Input: part model. Units: mm. Frame: model coordinates. A direction names the side the tool comes from. Give positions to 0.01 mm unless a question says otherwise; leave off trailing zeros. Order: outer loops, then holes, each group sorted by start corner. A loop starts at its lowest first (then second) coordinate and runs counter-clockwise, first axis right, second up. Notation, with made-up numbers: M 88,-37.5 L 109,-37.5 A24 ccw 109,-12.5 Z; hole C 19,8 d2. An arc over 180 degrees is marked long. Use a Markdown table: item, result.
Autodesk Inventor part; units mm, degrees
ref_plane "YZ Plane" through (0, 0, 0) normal (1, 0, 0) x (0, 1, 0)
ref_plane "XZ Plane" through (0, 0, 0) normal (0, 1, 0) x (-1, 0, 0)
ref_plane "XY Plane" through (0, 0, 0) normal (0, 0, 1) x (1, 0, 0)
sketch "Sketch1" plane through (0, 0, 0) normal (1, 0, 0) x (0, 1, 0)
  line L0 (-22.6931, 110) -> (55.0359, 110)
  line L1 (55, -110) -> (-22.6931, -110)
  line L2 (-62.7298, 0) -> (-22.6931, -110)
  line L3 (-62.7298, 0) -> (-22.6931, 110)
  line L4 (-57.4089, 0) -> (-19.449, -104.2938)
  line L5 (-14.4482, -105) -> (55, -105)
  line L6 (55.0359, 105) -> (-14.4122, 105)
  line L7 (-19.449, 104.2938) -> (-57.4089, 0)
  line L8 (55.0034, 17.6855) -> (-14.4593, 17.6855)
  line L9 (55.0034, 22.5) -> (-14.4456, 22.5496)
  line L10 (55, -52.5) -> (-14.449, -52.5)
  line L11 (55, -47.6855) -> (-14.449, -47.7352)
  line L12 (-60.6224, -5.7899) -> (-60, -7.5)
  line L13 (-60.6224, 5.7899) -> (-60, 7.5)
  line L14 (-14.4122, 105) -> (-14.4122, 68.1255)
  line L15 (-14.4456, 59.4672) -> (-14.4456, 22.5496)
  line L16 (-19.449, 104.2938) -> (-19.449, 68.1255)
  line L17 (-14.4593, 17.6855) -> (-14.4593, -10.5317)
  line L18 (-14.449, -19.4683) -> (-14.449, -47.7352)
  line L19 (-19.4705, 59.4672) -> (-19.4705, -10.5317)
  line L20 (-14.449, -52.5) -> (-14.449, -74.4672)
  line L21 (-14.4482, -83.1255) -> (-14.4482, -105.0928)
  line L22 (-19.4499, -19.4683) -> (-19.4499, -74.4672)
  line L23 (-19.449, -83.1255) -> (-19.449, -104.2938)
  line L24 (-19.449, -74.4672) -> (-19.4499, -74.4672)
  line L25 (-14.4593, -83.1255) -> (-14.4482, -83.1255)
  line L26 (-19.4499, -19.4683) -> (-19.449, -19.4683)
  line L27 (-19.4705, -10.5317) -> (-19.449, -10.5317)
  line L28 (-14.4122, 68.1255) -> (-14.4125, 68.1255)
  line L29 (-19.4705, 59.4672) -> (-19.449, 59.4672)
  line L30 (55.0359, 105) -> (55.0359, 110)
  line L31 (55.0034, 22.5) -> (55.0034, 17.6855)
  line L32 (55, -47.6855) -> (55, -52.5)
  line L33 (55, -105) -> (55, -110)
  line L34 (-19.449, -91.3967) -> (-19.449, 76.5553)
  line L35 (-14.4122, 69.213) -> (-14.4225, 22.5496)
  line L36 (-14.4236, 17.6855) -> (-14.438, -47.7351)
  line L37 (-14.439, -52.5) -> (-14.4482, -94.1091)
  point P0 (0, 0)
extrude "Extrusion1" add sketch "Sketch1" along normal blind 160
sketch "Sketch2" plane through (0, -14.4236, 17.6855) normal (0, 1, -0.0002) x (1, 0, 0)
  circle A0 centre (80, 33.4744) radius 10
  circle A1 centre (80, 98.5003) radius 10
  circle A2 centre (80, -44.9284) radius 10
  point P0 (0, 17.6824)
  dimension "d24" = 20
  dimension "d25" = 20
  dimension "d26" = 20
extrude "Extrusion2" cut sketch "Sketch2" against normal blind 6
sketch "Sketch3" plane through (0, -22.6931, -110) normal (0, -0.9397, -0.342) x (1, 0, 0)
  point P0 (0, 95.6047)
sketch "Sketch4" plane through (0, -22.6931, -110) normal (0, -0.9397, -0.342) x (1, 0, 0)
  line L0 (0, 117.1568) -> (160, 117.1568)
  circle A0 centre (80, 117.1568) radius 7.5
  point P0 (0, 95.6047)
  dimension "d29" = 15
extrude "Extrusion3" cut sketch "Sketch4" against normal blind 10
sketch "Sketch5" plane through (0, 0, 0) normal (-1, 0, 0) x (0, 0, 1)
  line L0 (-110, -22.6931) -> (-110, 55)
  line L1 (-110, 55) -> (109.7253, 55)
  line L2 (109.7253, 55) -> (109.7253, -62.9244)
  line L3 (109.7253, -62.9244) -> (-110, -62.9244)
  line L4 (-110, -62.9244) -> (-110, 55)
  point P0 (0, 0)
extrude "Extrusion4" add sketch "Sketch5" along normal blind 5
sketch "Sketch6" plane through (160, 0, 0) normal (1, 0, 0) x (0, 0, -1)
  line L0 (-109.7253, 55) -> (-109.7253, -22.793)
  line L1 (110, -22.6931) -> (110, -62.9244)
  line L2 (-109.7253, 55) -> (110, 55)
  line L3 (110, 55) -> (110, -62.9244)
  line L4 (110, -62.9244) -> (-109.7253, -62.9244)
  line L5 (-109.7253, -62.9244) -> (-109.7253, 55)
  point P0 (0, 0)
extrude "Extrusion5" add sketch "Sketch6" along normal blind 5
sketch "Sketch7" plane through (0, -62.9244, 109.7253) normal (0, 0, 1) x (1, 0, 0)
  line L0 (-5, 117.9244) -> (165, 117.9244)
  line L1 (-5, 117.9244) -> (165, 117.9244)
  line L2 (165, 117.9244) -> (165, 0)
  line L3 (165, 0) -> (-5, 0)
  line L4 (-5, 0) -> (-5, 117.9244)
  line L5 (165, 0) -> (-5, 0)
  line L6 (-5, 0) -> (-5, 117.9244)
  line L7 (-5, 117.9244) -> (165, 117.9244)
  line L8 (165, 117.9244) -> (165, 0)
  point P0 (0, 62.9244)
sketch "Sketch8" plane through (0, -22.6931, 110) normal (0, -0.9397, 0.342) x (1, 0, 0)
  circle A0 centre (144.5406, -21.5508) radius 6.0469
  point P0 (0, -95.6047)
extrude "Extrusion6" cut sketch "Sketch8" against normal blind 6
sketch "Sketch9" plane through (0, -62.9244, -110) normal (0, 0, -1) x (-1, 0, 0)
  line L0 (-165, 117.9244) -> (-165, 0)
  line L1 (0, 117.9244) -> (5, 117.9244)
  line L2 (-165, 0) -> (5, 0)
  line L3 (5, 0) -> (5, 117.9244)
  line L4 (5, 117.9244) -> (-165, 117.9244)
  line L5 (-165, 117.9244) -> (-165, 0)
  point P0 (0, 62.9244)
extrude "Extrusion7" add sketch "Sketch9" along normal blind 5
properties part number "Storage Tank"
1) Cut plane A-A on y = -42.5. Return loops of the section in (x, z).
Response values:
| item | result |
|---|---|
| outline | M -5,-115 L 165,-115 L 165,109.73 L 160,109.73 L 160,55.58 L 0,55.58 L 0,109.73 L -5,109.73 Z; hole M 0,-110 L 160,-110 L 160,-55.58 L 0,-55.58 Z; hole M 0,-40.96 L 160,-40.96 L 160,40.96 L 0,40.96 Z |
2) Cut plane B-B on z = 32.5. Return loops of the section in (x, y).
Response values:
| item | result |
|---|---|
| outline | M -5,-62.92 L 0,-62.92 L 0,-50.9 L 160,-50.9 L 160,-62.92 L 165,-62.92 L 165,55 L 160,55 L 160,-14.42 L 0,-14.42 L 0,55 L -5,55 Z; hole M 0,-45.58 L 160,-45.58 L 160,-19.45 L 0,-19.45 Z |
3) First-contact query: pin 1 Ø16 at (x, z) = (80, 62.61) entering from +Y; pin 2 Ø1.5 at (x, z) = (-3.5, 53) entering from +Y; pin 3 Ø6.5 at (x, z) = (90.5, 74.5) entering from -Y. Flat tips, straight axial feed; report the tip coordinate or a pass-through.
Response values:
| item | result |
|---|---|
| pin 1 | stops at y = -31.71 |
| pin 2 | stops at y = 55 |
| pin 3 | stops at y = -36.8 |
4) Reachability of faces 4 (the face through (81, -43, -110)), 5 (the face through (78.9, -38.7, -51.4)), 6 (the face through (160, 21, -15)) from +Z, -Z, +X, -X, +Y, -Y: full face, straight path, thin tool, end or side. Return the list, or none.
Response values:
| item | result |
|---|---|
| face 4 | -Y |
| face 5 | none |
| face 6 | +Y |
5) Material intervals for line 1 (Z direction, x = 80, y = -15); line 2 (Z direction, x = 79, y = -18.5); line 3 (X direction, y = -29.5, z = 21.5), sorted ascending. Write a range as from..to.
Response values:
| item | result |
|---|---|
| line 1 | z = -115..-90.81, -70.81..-25.79, -5.79..52.61, 72.61..110 |
| line 2 | z = -115..-90.76, -70.86..-25.74, -5.84..52.66, 72.56..110 |
| line 3 | x = -5..0, 160..165 |
6) Mould query, pull axis Y, two halves, no side actions, for faces 1 (the face through (79, 16, 110)), 2 (the face through (79, 55.036, 107)), 3 (the face through (0, -34, -1)). Classes: released by +Y, released by -Y, zero draft, split by the parting line, or undercut.
Response values:
| item | result |
|---|---|
| face 1 | zero draft |
| face 2 | released by +Y |
| face 3 | undercut |
